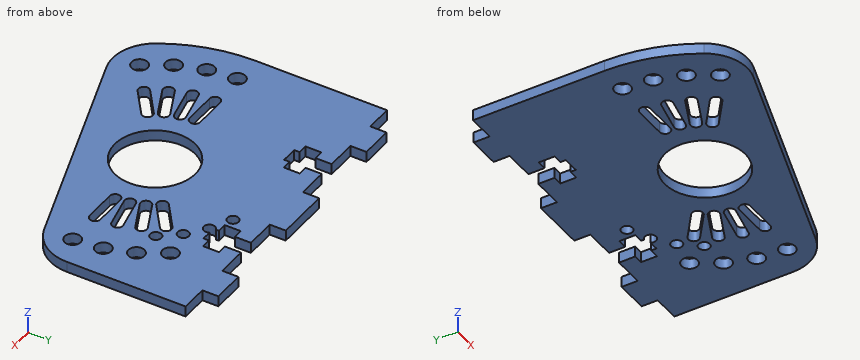
```python
from build123d import *

# Parameters (mm, degrees)
SKETCH_1_W               = 61.5
SKETCH_1_H               = 55
SKETCH_1_R               = 7.5
EXTRUDE_1_DEPTH          = 2
SKETCH_2_R               = 1.5
SKETCH_2_R_2             = 1.05
CUT_EXTRUDE_1_DEPTH      = 42.301483024
PATTERN_CIRCULAR_1_COUNT = 4
PATTERN_CIRCULAR_1_ANGLE = 37.5
CUT_EXTRUDE_2_DEPTH      = 42.301483024
FILLET_1_R               = 8
SKETCH_5_W               = 5
SKETCH_5_H               = 3
CUT_EXTRUDE_3_DEPTH      = 41.930581622


with BuildPart() as part:
    # 草图1 → 凸台-拉伸1 (new body)
    with BuildSketch(Plane.XY):
        Rectangle(SKETCH_1_W, SKETCH_1_H)
        Circle(SKETCH_1_R, mode=Mode.SUBTRACT)
    extrude(amount=EXTRUDE_1_DEPTH)

    # 草图2 → 切除-拉伸1 (cut, through all)
    with BuildSketch(Plane.XY.offset(2)):
        with Locations((24.75, 0)):
            Circle(SKETCH_2_R)
        with Locations((-24.75, 0)):
            Circle(SKETCH_2_R)
        with Locations((17.06, 10.73)):
            Circle(SKETCH_2_R_2)
        with BuildLine():
            Line((-18, 1), (-12, 1))
            ThreePointArc((-12, 1), (-11, 0), (-12, -1))
            Line((-12, -1), (-18, -1))
            ThreePointArc((-18, -1), (-19, 0), (-18, 1))
        make_face()
        with BuildLine():
            Line((12, 1), (18, 1))
            ThreePointArc((18, 1), (19, 0), (18, -1))
            Line((18, -1), (12, -1))
            ThreePointArc((12, -1), (11, 0), (12, 1))
        make_face()
    cut_extrude_1 = extrude(amount=-CUT_EXTRUDE_1_DEPTH, mode=Mode.SUBTRACT)

    # 阵列(圆周)1: 切除-拉伸1 ×4 about axis
    pattern_circular_1_axis = Axis((0, 0, 0), (0, 0, 1))
    for i in range(1, PATTERN_CIRCULAR_1_COUNT):
        add(cut_extrude_1.rotate(pattern_circular_1_axis, i * PATTERN_CIRCULAR_1_ANGLE / (PATTERN_CIRCULAR_1_COUNT - 1)), mode=Mode.SUBTRACT)

    # 草图3 → 切除-拉伸2 (cut, through all)
    with BuildSketch(Plane.XY.offset(2)):
        with BuildLine():
            Line((-21.720093373, -21.05469173), (30.048992854, -3.481454933))
            ThreePointArc((30.048992854, -3.481454933), (30.199706405, -1.743626417), (30.25, 0))
            Line((30.25, 0), (30.25, 27.5))
            Line((30.25, 27.5), (30.75, 27.5))
            Line((30.75, 27.5), (30.75, 0))
            Line((30.75, 0), (30.75, -27.5))
            Line((30.75, -27.5), (-30.75, -27.5))
            Line((-30.75, -27.5), (-30.75, 0))
            Line((-30.75, 0), (-30.75, 27.5))
            Line((-30.75, 27.5), (-30.25, 27.5))
            Line((-30.25, 27.5), (-30.25, 0))
            ThreePointArc((-30.25, 0), (-28.036541553, -11.358469867), (-21.720093373, -21.05469173))
        make_face()
    extrude(amount=-CUT_EXTRUDE_2_DEPTH, mode=Mode.SUBTRACT)

    # 圆角1
    fillet_1_edges = [part.edges().sort_by_distance(p)[0] for p in [
        (30.048992854, -3.481454933, 1),
        (-21.720093373, -21.05469173, 1),
    ]]
    fillet(fillet_1_edges, radius=FILLET_1_R)

    # 草图5 → 切除-拉伸3 (cut, through all)
    with BuildSketch(Plane.XY.offset(2)):
        with Locations((-27.75, 26)):
            Rectangle(SKETCH_5_W, SKETCH_5_H)
        Polygon((-19.25, 27.5), (-5, 27.5), (-5, 24.5), (-10.625, 24.5), (-10.625, 21.5), (-8.875, 21.5), (-8.875, 18.5), (-10.625, 18.5), (-10.625, 17.5), (-13.625, 17.5), (-13.625, 18.5), (-15.375, 18.5), (-15.375, 21.5), (-13.625, 21.5), (-13.625, 24.5), (-19.25, 24.5), align=None)
        Polygon((5, 27.5), (19.25, 27.5), (19.25, 24.5), (13.625, 24.5), (13.625, 21.5), (15.375, 21.5), (15.375, 18.5), (13.625, 18.5), (13.625, 17.5), (10.625, 17.5), (10.625, 18.5), (8.875, 18.5), (8.875, 21.5), (10.625, 21.5), (10.625, 24.5), (5, 24.5), align=None)
        with Locations((27.75, 26)):
            Rectangle(SKETCH_5_W, SKETCH_5_H)
    extrude(amount=-CUT_EXTRUDE_3_DEPTH, mode=Mode.SUBTRACT)


solid = part.part
```
Read the model definition and answer for the solid it produces. Units are mm, in the model's axes. Coordinates: 2 decimals unless noted, no trailing zeros. Loops run counter-clockwise (first coordinate to the right, second up) from the corner with the lowest first, then second, coordinate; pieces in that order, holes last. Notation, with made-up numbers: (12, 50.25) -> (23, 50.25) arc R10 ccw to (23, 67.25) -> close; hole circle Ø1 at (75, 67). An arc over 180 degrees is marked (long way). Return JSON: item names as keys, results as strings.
Item 1: Find the intervals of material crossed by probe 1 along X at (y, z) = (21, 0.15) (3 decimals); probe 2 along X at (y, z) = (22, 0.2) (3 decimals); probe 3 along Y at (x, z) = (23.5, 1.6), in increasing order.
Answers:
{"probe 1": "x = -30.25 to -15.375, -8.875 to 8.875, 15.375 to 30.25", "probe 2": "x = -30.25 to -13.625, -10.625 to 10.625, 13.625 to 30.25", "probe 3": "y = -5.7 to -0.83, 0.83 to 4.01, 6.7 to 9.41, 11.51 to 27.5"}
Item 2: Flat-ended cylindrical pins translate along their axes: P1, Ø1, axis at y = 25.5, z = 1, coming from the -X side; P2, Ø0.9, axis at x = 14.5, z = 1, coming from the +Y side; P3, Ø1, axis at x = -8.5, z = 0.5, coming from the -Y side. Find the tip coordinate at first contact, or state that the pin passes through.
Answers:
{"P1": "stops at x = -25.25", "P2": "stops at y = 24.5", "P3": "stops at y = -16.74"}
Item 3: Find section B-B (z = 1.4). Count the separate pieces of the cut face and the enclosed holes in it, plus the area to 3 significant figures.
Answers:
{"separate pieces": "1", "enclosed holes": "20", "area": "1,860 mm2"}
Item 4: Find section A-A (x = -13). Determine the outline of the cut face in (y, z).
Answers:
{"outline": "(-18.09, 0) -> (-11.24, 0) -> (-11.24, 2) -> (-18.09, 2) -> close; (-8.71, 0) -> (-7.17, 0) -> (-7.17, 2) -> (-8.71, 2) -> close; (-4.96, 0) -> (-3.91, 0) -> (-3.91, 2) -> (-4.96, 2) -> close; (-1.86, 0) -> (-1, 0) -> (-1, 2) -> (-1.86, 2) -> close; (1, 0) -> (17.5, 0) -> (17.5, 2) -> (1, 2) -> close"}
